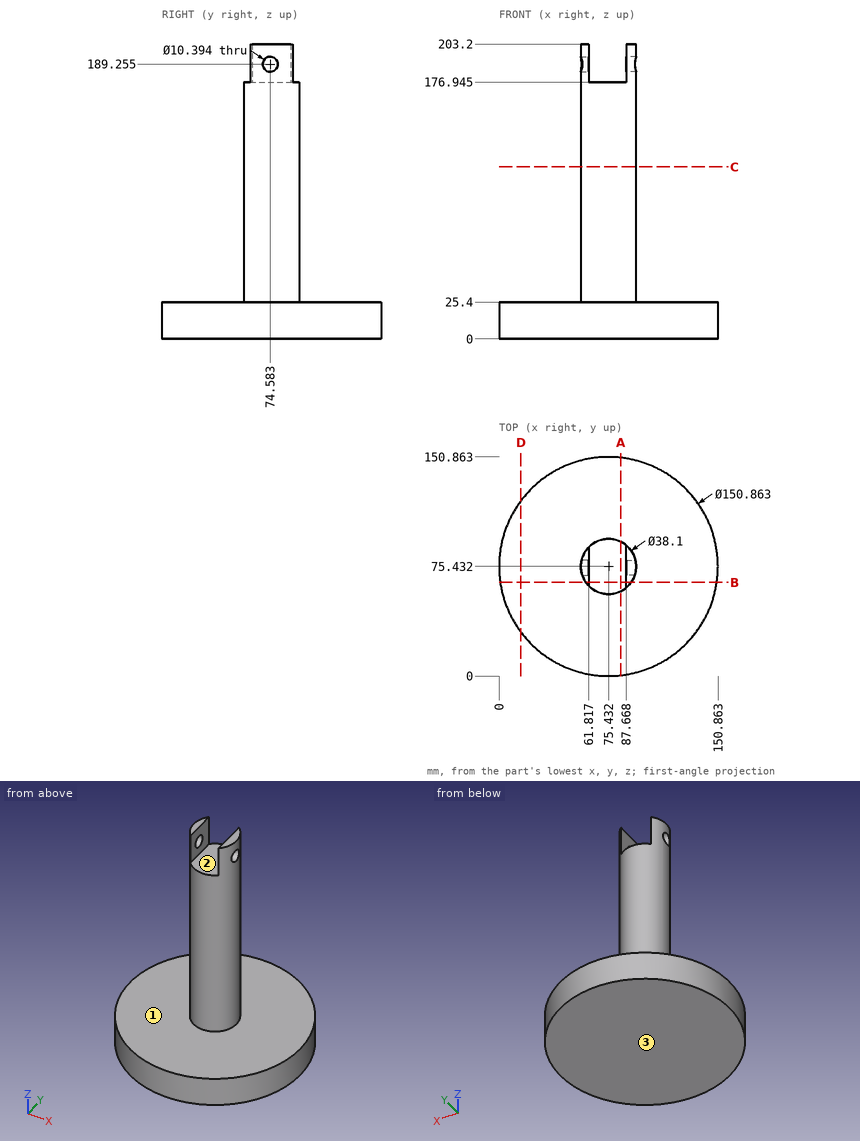
Job drawing, mm, ordinate dimensions from the low corner. One solid piece. A direction names the side the tool comes from. Coordinates: 2 decimals unless noted, no trailing zeros. Write each loop counter-clockwise with the first axis right and the second up, starting at its lowest first coordinate (ties: lowest second). Pieces come first, ordered by that corner, then holes.
Item 1: Slice it at C-C (z = 118.5). Write the cut outline in (x, y).
Item 2: Which spindle directions (+Z, -Z, +X, -X, +Y, -Y) get a long thin tool onto all of the face, cutting with end or side? Do the marked faces 1, 2 and 3. Say none if no direction does.
Item 3: Slice it at B-B (y = 64.5). Write the cut outline in (x, z) (1 decimal), and give its area (3 significant figures).
Item 4: Slice it at D-D (x = 15). Write the cut outline in (y, z) (1 decimal).
Item 5: Probe line 1 (Z direction, x = 12.5, y = 59); line 2 (Y direction, x = 81.5, z = 138.5) (1 decimal); line 3 (Y direction, x = 45, z = 14). List the from-to ranges inside material, lowest first.
Item 6: Slice it at A-A (x = 84). Write the cut outline in (y, z) (1 decimal).
Item 7: Pin check, flat tips, straight feed: pin 1 (20.5 mm diameter, centred on x = 72, y = 72.5, fed in from +Z); pin 2 (8 mm diameter, centred on x = 101.5, z = 82.5, fed in from +Y); pin 3 (8 mm diameter, centred on y = 68, z = 192, fed in from -X) (1 decimal); pin 4 (10 mm diameter, centred on x = 65, z = 66.5, fed in from +Y). Stop position of each tip, or through.
Results found:
1. outline: circle Ø38.1 at (75.43, 75.43)
2. face 1: +Z
2. face 2: +Z, +Y, -Y
2. face 3: -Z, +X, -X, +Y, -Y
3. outline: (0.8, 0) - (150.1, 0) - (150.1, 25.4) - (91, 25.4) - (91, 203.2) - (87.7, 203.2) - (87.7, 176.9) - (61.8, 176.9) - (61.8, 203.2) - (59.8, 203.2) - (59.8, 25.4) - (0.8, 25.4) - close
3. area: 8,660 mm2
4. outline: (30.3, 0) - (120.6, 0) - (120.6, 25.4) - (30.3, 25.4) - close
5. line 1: z = 0 to 25.4
5. line 2: y = 57.4 to 93.5
5. line 3: y = 6.41 to 144.45
6. outline: (0.5, 0) - (150.4, 0) - (150.4, 25.4) - (92.4, 25.4) - (92.4, 176.9) - (58.4, 176.9) - (58.4, 25.4) - (0.5, 25.4) - close
7. pin 1: stops at z = 203.2
7. pin 2: passes through
7. pin 3: stops at x = 56.8
7. pin 4: stops at y = 93.69
